Verification items for the finished model (mm, model axes). Give positions to 0.01 mm unless a question says otherwise; leave off trailing zeros. Order: outer loops, then holes, each group sorted by start corner. A loop starts at its lowest first (then second) coordinate and runs counter-clockwise, first axis right, second up. Notation, with made-up numbers: (-37.75, 40) -> (-32.75, 40) arc R13 ccw to (-32.75, 46) -> close; hole circle Ø4 at (-29.5, 4). An arc over 180 degrees is marked (long way). Write each question's results on one line, items separated by ' | '. Start each with the question number.
1. Cross-section at A-A, the plane x = 0. Enter the section's corners in (y, z).
2. Depth check by flat-ended pin: pin 1 Ø2.5 at (y, z) = (41, 11.5) entering from +X; pin 2 Ø6 at (y, z) = (-15, 4.5) entering from -X; pin 3 Ø1.5 at (y, z) = (41, 13) entering from +X. Enter the tip coordinate at first touch or a pass-through.
3. Cross-section at D-D, the plane y = -33. Enter the section's corners in (x, z), then the cut area to 3 significant figures.
4. Cross-section at C-C, the plane z = 13. State how many separate pieces and enclosed holes the cut face has, then the cut area to 3 significant figures.
5. Cross-section at B-B, the plane z = 4.75. Enter the section's corners in (x, y), then the cut area to 3 significant figures.
6. Material ranges on L1, parallel to X at y = 39.5, z = 10.75; L2, parallel to X at y = -42, z = 11.5; L3, parallel to Y at x = 0, z = 13.35, recorded low to high. Write a range as from..to.
from build123d import *

# Parameters (mm, degrees)
F1_DEPTH = 15
F2_SIZE  = 25
F3_W     = 15
F3_H     = 5
F4_DEPTH = 5
F5_R     = 5.5
F6_DEPTH = 5


with BuildPart() as f1:
    # F0 (on Top) → F1 (new body)
    with BuildSketch(Plane.XY):
        Polygon((-77.942286, 45), (0, -90), (77.942286, 45), align=None)
    extrude(amount=F1_DEPTH)

    # F2
    f2_edges = [f1.edges().sort_by_distance(p)[0] for p in [
        (0, -90, 7.5),
        (77.942286, 45, 7.5),
        (-77.942286, 45, 7.5),
    ]]
    chamfer(f2_edges, length=F2_SIZE)

    # F3 (on face) → F4 (cut)
    with BuildSketch(Plane.XY.offset(15)):
        with Locations((-17.5, 40)):
            Rectangle(F3_W, F3_H)
        with Locations((17.5, 40)):
            Rectangle(F3_W, F3_H)
        Polygon((41.80608, -12.589746), (49.30608, 0.400635), (44.975953, 2.900635), (37.475953, -10.089746), align=None)
        Polygon((31.80608, -29.910254), (27.475953, -27.410254), (19.975953, -40.400635), (24.30608, -42.900635), align=None)
        Polygon((-31.80608, -29.910254), (-24.30608, -42.900635), (-19.975953, -40.400635), (-27.475953, -27.410254), align=None)
        Polygon((-41.80608, -12.589746), (-37.475953, -10.089746), (-44.975953, 2.900635), (-49.30608, 0.400635), align=None)
    extrude(amount=-F4_DEPTH, mode=Mode.SUBTRACT)

    # F5 (on face) → F6 (cut)
    with BuildSketch(Plane.XY.offset(15)):
        with Locations((0, -53.349365)):
            Circle(F5_R)
        with Locations((-46.201905, 26.674682)):
            Circle(F5_R)
        with Locations((46.201905, 26.674682)):
            Circle(F5_R)
    extrude(amount=-F6_DEPTH, mode=Mode.SUBTRACT)


solid = f1.part
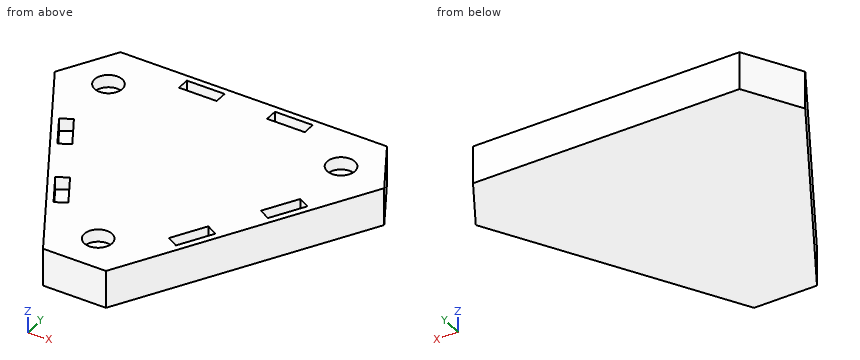
Results below:
1) outline: (-68.35, 0) -> (45, 0) -> (45, 15) -> (-47.85, 15) -> (-47.85, 10) -> (-58.85, 10) -> (-58.85, 15) -> (-68.35, 15) -> close
2) pin 1: stops at x = 55.97 | pin 2: stops at x = -45.03 | pin 3: stops at x = 55.68
3) outline: (-32.91, 0) -> (32.91, 0) -> (32.91, 15) -> (30.02, 15) -> (30.02, 10) -> (24.25, 10) -> (24.25, 15) -> (-24.25, 15) -> (-24.25, 10) -> (-30.02, 10) -> (-30.02, 15) -> (-32.91, 15) -> close | area: 930 mm²
4) separate pieces: 1 | enclosed holes: 9 | area: 8,980 mm²
5) outline: (-65.44, 23.35) -> (-12.5, -68.35) -> (12.5, -68.35) -> (65.44, 23.35) -> (52.94, 45) -> (-52.94, 45) -> close | area: 9,710 mm²
6) L1: x = -56.12..-25, -10..10, 25..56.12 | L2: x = -27.71..-24.83, -22.75..22.75, 24.83..27.71 | L3: y = -68.35..-58.85, -47.85..45
